Can you work these out from the model? Positions are in its coordinate system, mm. A direction names the side the tool comes from. Give positions to 0.01 mm unless a question says otherwise; leave off trailing zeros. Loops run counter-clockwise (first coordinate to the right, second up) from the corner with the lowest first, then second, coordinate; pieces in that order, holes last. Notation, with made-up numbers: M 47.25,-24.75 L 74.25,-24.75 A16 cw 74.25,-3.75 Z; hole C -15,80.5 d10. An arc over 180 degrees is marked long. Use CSV: the item, a comma, the result in double quotes.
from build123d import *

# Parameters (mm, degrees)
F0_W     = 10.3
F0_H     = 20
F0_W_2   = 2.7
F1_DEPTH = 2.5
F2_DEPTH = 32.5
F4_D     = 18.75
F5_D     = 3.7
F6_DEPTH = 5
F7_SIZE2 = 9
F7_SIZE  = 5
F8_R     = 10
F9_R     = 3
F10_R    = 1


with BuildPart() as f1:
    # F0 (on Front) → F1 (new body)
    with BuildSketch(Plane.XZ):
        Polygon((13.0521883406, 19.9863334329), (-17.9478116594, 19.9863334329), (-17.9478116594, 7.9863334329), (-7.6478116594, 7.9863334329), (-4.9478116594, 7.9863334329), (0.0521883406, 7.9863334329), (0.0521883406, 11.4863334329), (4.0521883406, 11.4863334329), (4.0521883406, 7.9863334329), (13.0521883406, 7.9863334329), align=None)
        Polygon((-17.9478116594, -50.0136665671), (-17.9478116594, -40.1987119909), (-34.9478116594, -50.0136665671), align=None)
        with Locations((-12.7978116594, -2.0136665671)):
            Rectangle(F0_W, F0_H)
        with Locations((-6.2978116594, -2.0136665671)):
            Rectangle(F0_W_2, F0_H)
        Polygon((-7.6478116594, -12.0136665671), (-17.9478116594, -12.0136665671), (-17.9478116594, -40.1987119909), (-17.9478116594, -50.0136665671), (-4.9478116594, -50.0136665671), (-4.9478116594, -12.0136665671), align=None)
    extrude(amount=F1_DEPTH)

    # F0 (on Front) → F2 (join)
    with BuildSketch(Plane.XZ):
        Polygon((-4.9478116594, -50.0136665671), (-17.9478116594, -50.0136665671), (-34.9478116594, -50.0136665671), (-34.9478116594, -52.5136665671), (-4.9478116594, -52.5136665671), align=None)
    extrude(amount=F2_DEPTH)

    # F4 (through all)
    with Locations(Plane.XY):
        with Locations((-19.9478116594, -17.5)):
            Hole(F4_D / 2)

    # F5 (through all)
    with Locations(Plane(origin=(0, 0, 0), x_dir=(1, 0, 0), z_dir=(0, 1, 0))):
        with Locations((-12.9478116594, -12.4863334329), (8.0521883406, -12.4863334329)):
            Hole(F5_D / 2)

    # F0 (on Front) → F6 (join)
    with BuildSketch(Plane.XZ):
        with Locations((-12.7978116594, -2.0136665671)):
            Rectangle(F0_W, F0_H)
    extrude(amount=-F6_DEPTH)

    # F7
    f7_edges = [f1.edges().sort_by_distance(p)[0] for p in [
        (-17.947812, 5, -2.013667),
    ]]
    f7_side = f1.faces().sort_by_distance((-17.947812, 0.247229, -6.875159))[0]
    chamfer(f7_edges, length=F7_SIZE, length2=F7_SIZE2, reference=f7_side)

    # F8
    f8_edges = [f1.edges().sort_by_distance(p)[0] for p in [
        (-4.947812, -32.5, -51.263667),
        (-34.947812, -32.5, -51.263667),
    ]]
    fillet(f8_edges, radius=F8_R)

    # F9
    f9_edges = [f1.edges().sort_by_distance(p)[0] for p in [
        (-17.947812, -1.25, 19.986333),
        (13.052188, -1.25, 19.986333),
        (0.052188, -1.25, 7.986333),
        (4.052188, -1.25, 7.986333),
        (13.052188, -1.25, 7.986333),
        (-19.947812, 0, -52.513667),
        (-19.947812, -2.5, -50.013667),
    ]]
    fillet(f9_edges, radius=F9_R)

    # F10
    f10_edges = [f1.edges().sort_by_distance(p)[0] for p in [
        (0.052188, -1.25, 11.486333),
        (4.052188, -1.25, 11.486333),
        (-4.947812, -1.25, 7.986333),
    ]]
    fillet(f10_edges, radius=F10_R)


solid = f1.part
Q1. I want a section at B-B, the plane x = -26. Please give me the cut outline in (y, z), then the cut area to 3 significant figures.
Model answer:
outline,"M -32.44,-52.51 L -24.66,-52.51 L -24.66,-50.01 L -32.44,-50.01 Z; M -10.34,-52.51 L -3,-52.51 A3 ccw 0,-49.51 L 0,-44.85 L -2.5,-44.85 L -2.5,-47.01 A3 cw -5.5,-50.01 L -10.34,-50.01 Z"
area,"58.2 mm2"
Q2. I'm going to push flat-ended pins straight in: P1, Ø12, axis at y = -10.5, z = 0.5, coming from the +X side; P2, Ø2, axis at y = -1, z = -7.5, coming from the -X side; P3, Ø2, axis at x = 8.5, y = -1.5, coming from the -Z side; P4, Ø2.5, axis at y = 2, z = -4, coming from the +X side. Where does each tip first touch, or does it pass through?
Model answer:
P1,"through"
P2,"x = -17.95"
P3,"z = 7.99"
P4,"x = -7.65"
Q3. I want a section at D-D, the plane x = -21. Please give me the cut outline in (y, z).
Model answer:
outline,"M -32.5,-52.51 L -26.82,-52.51 L -26.82,-50.01 L -32.5,-50.01 Z; M -8.18,-52.51 L -3,-52.51 A3 ccw 0,-49.51 L 0,-41.96 L -2.5,-41.96 L -2.5,-47.01 A3 cw -5.5,-50.01 L -8.18,-50.01 Z"
Q4. I want a section at C-C, the plane z = 15.5. Please give me the cut outline in (x, y).
Model answer:
outline,"M -17.95,-2.5 L 13.05,-2.5 L 13.05,0 L -17.95,0 Z"
Q5. Please list where these lines run through material, in increasing order: L1, parallel to X at y = -17, z = -51; L2, parallel to Z at x = -11, y = -31; L3, parallel to Y at x = -4, z = 17. Write a range as from..to.
Model answer:
L1,"-34.95..-29.31, -10.59..-4.95"
L2,"-52.51..-50.01"
L3,"-2.5..0"
Q6. For faces 5 (the cylindrical face through (5.091, -1.268, 8.716)), 6 (the flat face through (-8, -2.5, -13)), 7 (the cylindrical face through (12.2, -1.27, 8.89)), which set-ups out of +Z, -Z, +X, -X, +Y, -Y let a thin tool reach every point of the face, with its end or its side?
Model answer:
face 5,"-Z, +Y, -Y"
face 6,"+Z, +X, -X, -Y"
face 7,"-Z, +X, +Y, -Y"
Q7. If we mould it in two halves opening along X, with no side actions, what happens to faces 1 (the flat face through (-13.385, 2.535, -2.154)), 2 (the flat face through (2, -1, 11.486)), 3 (the cylindrical face through (-0.986, -1.268, 8.716)), 4 (the cylindrical face through (12.15, -1.27, 19.13))? For each: released by +X, released by -X, zero draft, split by the parting line, or undercut.
Model answer:
face 1,"released by -X"
face 2,"undercut"
face 3,"undercut"
face 4,"released by +X"
Q8. I want a section at A-A, the plane y = -17.5. Please give me the cut outline in (x, z), then the cut area to 3 significant figures.
Model answer:
outline,"M -34.95,-52.51 L -29.32,-52.51 L -29.32,-50.01 L -34.95,-50.01 Z; M -10.57,-52.51 L -4.95,-52.51 L -4.95,-50.01 L -10.57,-50.01 Z"
area,"28.1 mm2"
